from build123d import *

# Parameters (mm, degrees)
ESBO_O1_W                               = 90
ESBO_O1_H                               = 270
RESSALTO_EXTRUS_O1_DEPTH                = 10.7
FURO_ROSCADO_PARA_CONDU_TE_DE_M5X0_81_D = 5.2
FURO_ROSCADO_PARA_CONDU_TE_DE_1_4_281_D = 6.6294
FURO_ROSCADO_PARA_CONDU_TE_DE_M5X0_82_D = 5.2
FURO_ROSCADO_PARA_CONDU_TE_DE_10_321_D  = 5.1054
ESBO_O14_R                              = 11
CORTE_EXTRUS_O1_DEPTH                   = 11.7
FURO_ROSCADO_PARA_CONDU_TE_DE_M3X0_51_D = 3.15


with BuildPart() as part:
    # Esboço1 → Ressalto-extrusão1 (new body)
    with BuildSketch(Plane.XY):
        Rectangle(ESBO_O1_W, ESBO_O1_H)
    extrude(amount=RESSALTO_EXTRUS_O1_DEPTH)

    # Furo roscado para conduíte de M5x0.81 (through all)
    with Locations(Plane(origin=(0, 0, 0), x_dir=(-1, 0, 0), z_dir=(0, 0, -1))):
        with Locations((-40, -98.75), (-14, -98.75), (-40, -129.25), (-14, -129.25), (14, -129.25), (40, -129.25), (14, -98.75), (40, -98.75)):
            Hole(FURO_ROSCADO_PARA_CONDU_TE_DE_M5X0_81_D / 2)

    # Furo roscado para conduíte de 1/4-281 (through all)
    with Locations(Plane(origin=(0, 0, 0), x_dir=(-1, 0, 0), z_dir=(0, 0, -1))):
        with Locations((-20, -85), (20, -85)):
            Hole(FURO_ROSCADO_PARA_CONDU_TE_DE_1_4_281_D / 2)

    # Furo roscado para conduíte de M5x0.82 (through all)
    with Locations(Plane(origin=(0, 0, 0), x_dir=(-1, 0, 0), z_dir=(0, 0, -1))):
        with Locations((-35, 125), (-35, 20)):
            Hole(FURO_ROSCADO_PARA_CONDU_TE_DE_M5X0_82_D / 2)

    # Furo roscado para conduíte de #10-321 (through all)
    with Locations(Plane(origin=(0, 0, 0), x_dir=(-1, 0, 0), z_dir=(0, 0, -1))):
        with Locations((-5, 125), (-5, 89), (-5, 39), (-5, 3)):
            Hole(FURO_ROSCADO_PARA_CONDU_TE_DE_10_321_D / 2)

    # Esboço14 → Corte-extrusão1 (cut, through all)
    with BuildSketch(Plane(origin=(0, 0, 0), x_dir=(-1, 0, 0), z_dir=(0, 0, -1))):
        with Locations((-4, 64)):
            Circle(ESBO_O14_R)
    extrude(amount=-CORTE_EXTRUS_O1_DEPTH, mode=Mode.SUBTRACT)

    # Furo roscado para conduíte de M3x0.51 (through all)
    with Locations(Plane(origin=(0, 0, 0), x_dir=(-1, 0, 0), z_dir=(0, 0, -1))):
        with Locations((-19.5, 79.5), (-19.5, 48.5), (11.5, 79.5), (11.5, 48.5)):
            Hole(FURO_ROSCADO_PARA_CONDU_TE_DE_M3X0_51_D / 2)


solid = part.part
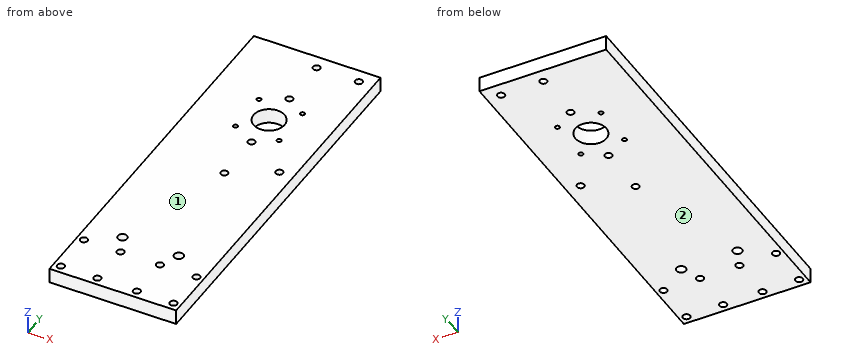
Geometry: final body of the model. Coordinates: model frame, mm. Face numbers are marked on the shaded views. Round coordinates to 2 decimals unless told otherwise and drop trailing zeros. Loops run counter-clockwise (first coordinate to the right, second up) from the corner with the lowest first, then second, coordinate; pieces in that order, holes last. Notation, with made-up numbers: (-1.5, 87.25) - (36.5, 87.25) arc R28 ccw to (36.5, 121.25) - close; hole circle Ø6 at (46, 73). An arc over 180 degrees is marked (long way). Write each question's results on one line, items separated by ' | '. Start each with the question number.
1) Cut plane B-B on x = 35. Return loops of the section in (y, z), then the cut area to 3 significant figures.
2) Mould query, pull axis Z, two halves, no side actions, for the marked faces 1 and 2. Classes: released by +Z, released by -Z, zero draft, split by the parting line, or undercut.
3) Cut plane D-D on z = 4. Count the separate pieces of the cut face and the enclosed holes in it, then the cut area to 3 significant figures.
4) First-contact query: P1, Ø6, axis at x = 35, y = 20, coming from the +Z side; P2, Ø4.5, axis at x = 14, y = -98.75, coming from the +Z side. Flat tips, straight axial feed; report the tip coordinate or a pass-through.
5) Cut plane A-A on y = 64. Return loops of the section in (x, z), then the cut area to 3 significant figures.
6) Cut plane C-C on y = -85. Return loops of the section in (x, z).
7) Line query: probe 1 along Y at (x, z) = (5, 3.75); probe 2 along X at (y, z) = (79.5, 9.25) (3 decimals); probe 3 along Y at (x, z) = (4, 8.5). Output: solid intervals per line, ascending. Write a range as [from, to].
Verdict:
1) outline: (-135, 0) - (17.4, 0) - (17.4, 10.7) - (-135, 10.7) - close; (22.6, 0) - (122.4, 0) - (122.4, 10.7) - (22.6, 10.7) - close; (127.6, 0) - (135, 0) - (135, 10.7) - (127.6, 10.7) - close | area: 2,780 mm2
2) face 1: released by +Z | face 2: released by -Z
3) separate pieces: 1 | enclosed holes: 21 | area: 23,500 mm2
4) P1: stops at z = 10.7 | P2: passes through
5) outline: (-45, 0) - (-7, 0) - (-7, 10.7) - (-45, 10.7) - close; (15, 0) - (45, 0) - (45, 10.7) - (15, 10.7) - close | area: 728 mm2
6) outline: (-45, 0) - (-23.31, 0) - (-23.31, 10.7) - (-45, 10.7) - close; (-16.69, 0) - (16.69, 0) - (16.69, 10.7) - (-16.69, 10.7) - close; (23.31, 0) - (45, 0) - (45, 10.7) - (23.31, 10.7) - close
7) probe 1: y = [-135, 0.45], [5.55, 36.45], [41.55, 53.05], [74.95, 86.45], [91.55, 122.45], [127.55, 135] | probe 2: x = [-45, -13.075], [-9.925, 17.925], [21.075, 45] | probe 3: y = [-135, 0.65], [5.35, 36.65], [41.35, 53], [75, 86.65], [91.35, 122.65], [127.35, 135]
